from build123d import *

# Parameters (mm, degrees)
F0_W         = 50
F0_H         = 54
F1_DEPTH     = 25.4
F2_W         = 41.8139733374
F2_H         = 8.200337179
F3_DEPTH     = 50.8
F4_W         = 8.200337179
F4_H         = 19.0244916171
F5_DEPTH     = 25.4
F7_D         = 5.08
F8_R         = 2.54
F9_W         = 50
F9_H         = 19.05
F10_DEPTH    = 8.128
F11_W        = 33.5916
F11_H        = 8.128
F12_DEPTH    = 25.4
F15_D        = 5.08
F15_ON_F13_D = 5.08
F16_R        = 2.54


with BuildPart() as f1:
    # F0 (on Top) → F1 (new body)
    with BuildSketch(Plane.XY):
        with Locations((-25.227407366, 34.7650984749)):
            Rectangle(F0_W, F0_H)
    extrude(amount=F1_DEPTH)

    # F2 (on face) → F3 (cut)
    with BuildSketch(Plane.XY.offset(25.4)):
        with Locations((-29.3204206973, 11.8652670644)):
            Rectangle(F2_W, F2_H)
    extrude(amount=-F3_DEPTH, mode=Mode.SUBTRACT)

    # F4 (on face) → F5 (cut)
    with BuildSketch(Plane(origin=(-8.4134340286, 0, 0), x_dir=(0, -1, 0), z_dir=(-1, 0, 0))):
        with Locations((-11.8652670644, 15.8877541915)):
            Rectangle(F4_W, F4_H)
    extrude(amount=-F5_DEPTH, mode=Mode.SUBTRACT)

    # F7 (through all)
    with Locations(Plane.XY.offset(6.3755083829)):
        with Locations((-4.3204206973, 11.8652670644)):
            Hole(F7_D / 2)

    # F8
    f8_edges = [f1.edges().sort_by_distance(p)[0] for p in [
        (-8.413434, 7.765098, 3.187754),
        (-0.227407, 7.765098, 3.187754),
    ]]
    fillet(f8_edges, radius=F8_R)

    # F9 (on face) → F10 (cut)
    with BuildSketch(Plane(origin=(0, 61.7650984749, 0), x_dir=(-1, 0, 0), z_dir=(0, 1, 0))):
        with Locations((25.227407366, 15.875)):
            Rectangle(F9_W, F9_H)
    extrude(amount=-F10_DEPTH, mode=Mode.SUBTRACT)

    # F11 (on face) → F12 (cut)
    with BuildSketch(Plane.XY.offset(6.35)):
        with Locations((-25.227407366, 57.7010984749)):
            Rectangle(F11_W, F11_H)
    extrude(amount=-F12_DEPTH, mode=Mode.SUBTRACT)

    # F15 (through all)
    with Locations(Plane.XY.offset(6.35)):
        with Locations((-4.329507366, 57.7010984749)):
            Hole(F15_D / 2)

    # F15 on F13 (through all)
    with Locations(Plane.XY.offset(6.35)):
        with Locations((-46.125307366, 57.7010984749)):
            Hole(F15_ON_F13_D / 2)

    # F16
    f16_edges = [f1.edges().sort_by_distance(p)[0] for p in [
        (-50.227407, 61.765098, 3.175),
        (-42.023207, 61.765098, 3.175),
        (-8.431607, 61.765098, 3.175),
        (-0.227407, 61.765098, 3.175),
    ]]
    fillet(f16_edges, radius=F16_R)


solid = f1.part
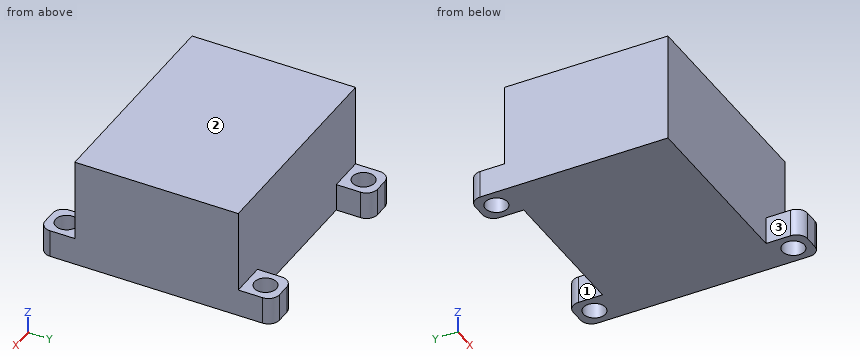
Here's how the part is built. I have some questions about the finished solid (model axes, mm). Face numbers are marked on the shaded views. A direction names the side the tool comes from. Round coordinates to 2 decimals unless told otherwise and drop trailing zeros. Loops run counter-clockwise (first coordinate to the right, second up) from the corner with the lowest first, then second, coordinate; pieces in that order, holes last. Notation, with made-up numbers: M -23,56 L 15,56 A15 ccw 15,72 Z; hole C 55.5,11.5 d4. An arc over 180 degrees is marked long. Write each question's results on one line, items separated by ' | '. Start each with the question number.
(1) I want a section at C-C (x = -34). Please give me the cut outline in (y, z), then the cut area to 3 significant figures.
(2) I want a section at A-A (x = -3.5). Please give me the cut outline in (y, z).
(3) I want a section at D-D (z = 15.5). Please give me the cut outline in (x, y), then the cut area to 3 significant figures.
(4) I want a section at B-B (z = 1.75). Please give me the cut outline in (x, y), then the cut area to 3 significant figures.
(5) If I drill on probe 1 along X at (y, z) = (12, 5); probe 2 along X at (y, z) = (57, 5.25); probe 3 along Y at (x, z) = (-46, 3.5), over which ranges is the centre line in solid material (lowest first)? Write a range as from..to.
(6) On a 3-axis mill with a long thin cutter (end or side, diameter ignored), from which of +Z, -Z, +X, -X, +Y, -Y can I reach the whole of each face in a straight line? I mean the marked faces 1, 2 and 3. Say none if no direction works.
(7) Will these pins go through, and if not, where does the flat tip stop? P1, Ø1, axis at x = -19.5, z = 12, coming from the +Y side; P2, Ø4.5, axis at y = 12.5, z = 4.5, coming from the -X side; P3, Ø8, axis at x = -46.13, y = 57.7, coming from the +Z side; P4, Ø4, axis at x = -4.33, y = 57.7, coming from the -Z side.
Solved:
1) outline: M 15.97,0 L 53.64,0 L 53.64,25.4 L 15.97,25.4 Z | area: 957 mm²
2) outline: M 7.77,0 L 9.46,0 L 9.46,6.38 L 7.77,6.38 Z; M 14.27,0 L 55.3,0 L 55.3,6.35 L 53.64,6.35 L 53.64,25.4 L 15.97,25.4 L 15.97,6.38 L 14.27,6.38 Z; M 60.1,0 L 61.77,0 L 61.77,6.35 L 60.1,6.35 Z
3) outline: M -50.23,15.97 L -0.23,15.97 L -0.23,53.64 L -50.23,53.64 Z | area: 1,880 mm²
4) outline: M -50.23,15.97 L -8.41,15.97 L -8.41,10.31 A2.54 ccw -5.87,7.77 L -2.77,7.77 A2.54 ccw -0.23,10.31 L -0.23,59.23 A2.54 ccw -2.77,61.77 L -5.89,61.77 A2.54 ccw -8.43,59.23 L -8.43,53.64 L -42.02,53.64 L -42.02,59.23 A2.54 ccw -44.56,61.77 L -47.69,61.77 A2.54 ccw -50.23,59.23 Z; hole C -46.13,57.7 d5.08; hole C -4.33,57.7 d5.08; hole C -4.32,11.87 d5.08 | area: 2,010 mm²
5) probe 1: x = -8.41..-6.86, -1.78..-0.23 | probe 2: x = -50.23..-48.57, -43.68..-42.02, -8.43..-6.77, -1.89..-0.23 | probe 3: y = 15.97..55.16, 60.24..61.77
6) face 1: +Z, -Z, +Y | face 2: +Z, +X, -X, +Y, -Y | face 3: +Z, -Z, -X, -Y
7) P1: stops at y = 53.64 | P2: stops at x = -8.41 | P3: stops at z = 6.35 | P4: passes through
